```python
from build123d import *

# Parameters (mm, degrees)
F3_R     = 11.3510766414
F4_DEPTH = 25.4
F0_R     = 13.8925555002
F0_R_2   = 11.3510766414
F5_R     = 11.3510766414
F6_DEPTH = 25.401


with BuildPart() as f4:
    # F3 (on face) → F4 (new body)
    with BuildSketch(Plane.XY):
        with Locations((-55.0634227693, 14.0889985487)):
            Circle(F3_R)
    extrude(amount=F4_DEPTH)

    # F5 (on face) → F6 (cut, through all)
    with BuildSketch(Plane.XY.offset(25.4)):
        with Locations((-55.0634227693, 14.0889985487)):
            Circle(F5_R)
    extrude(amount=-F6_DEPTH, mode=Mode.SUBTRACT)


with BuildPart() as f4b:
    # F0 (on Top) → F4, piece 2 (new body)
    with BuildSketch(Plane.XY):
        with Locations((-55.0634227693, 14.0889985487)):
            Circle(F0_R)
        with Locations((-55.0634227693, 14.0889985487)):
            Circle(F0_R_2, mode=Mode.SUBTRACT)
    extrude(amount=F4_DEPTH)


solid = f4b.part
```
Geometry: final body of the model. Coordinates: model frame, mm. Give positions to 0.01 mm unless a question says otherwise; leave off trailing zeros. Write each loop counter-clockwise with the first axis right and the second up, starting at its lowest first coordinate (ties: lowest second). Pieces come first, ordered by that corner, then holes.
1. Section query C-C, the plane z = 3.5. Return loops of the section in (x, y), then the cut area to 3 significant figures.
2. Draft query along Y for faces 1 (the cylindrical face through (-68.943, 14.7, 12.522)), 2 (the flat face through (-66.4, 16.2, 0)), 3 (the cylindrical face through (-49.826, 4.019, 12.522)). Return one class per face: released by +Y, released by -Y, zero draft, split by the parting line, or undercut.
3. Section query D-D, the plane x = -42.75. Return loops of the section in (y, z).
4. Section query A-A, the plane x = -53. Return loops of the section in (y, z), then the cut area to 3 significant figures.
5. Line query: probe 1 along X at (y, z) = (14.25, 8.75); probe 2 along Y at (x, z) = (-58.5, 9.5); probe 3 along X at (y, z) = (7.75, 23.5). Output: solid intervals per line, ascending.
6. Section query B-B, the plane y = 18. Return loops of the section in (x, z).
7. Pin query (flat end, axial travel): P1, Ø1.5, axis at y = 19, z = 19.5, coming from the -X side; P2, Ø1.5, axis at x = -52, z = 21, coming from the -Y side; P3, Ø4, axis at x = -61, z = 18.5, coming from the +Y side. Return the tip coordinate at first contact, or that it passes through.
Computed:
1. outline: circle Ø27.79 at (-55.06, 14.09); hole circle Ø22.7 at (-55.06, 14.09)
1. area: 202 mm2
2. face 1: split by the parting line
2. face 2: zero draft
2. face 3: undercut
3. outline: (7.66, 0) - (20.52, 0) - (20.52, 25.4) - (7.66, 25.4) - close
4. outline: (0.35, 0) - (2.93, 0) - (2.93, 25.4) - (0.35, 25.4) - close; (25.25, 0) - (27.83, 0) - (27.83, 25.4) - (25.25, 25.4) - close
4. area: 131 mm2
5. probe 1: x = -68.96 to -66.41, -43.71 to -41.17
5. probe 2: y = 0.63 to 3.27, 24.91 to 27.55
5. probe 3: x = -67.43 to -64.48, -45.65 to -42.7
6. outline: (-68.39, 0) - (-65.72, 0) - (-65.72, 25.4) - (-68.39, 25.4) - close; (-44.41, 0) - (-41.73, 0) - (-41.73, 25.4) - (-44.41, 25.4) - close
7. P1: stops at x = -68.32
7. P2: stops at y = 0.39
7. P3: stops at y = 27.41
